from build123d import *

# Parameters (mm, degrees)
SKETCH_1_W                   = 35
SKETCH_1_H                   = 150
EXTRUDE_1_DEPTH              = 4
HOLE_WIZARD_M3_1_D           = 3.4
HOLE_WIZARD_M3_1_CSINK_D     = 6.72
HOLE_WIZARD_M3_1_CSINK_ANGLE = 90


with BuildPart() as part:
    # 草图1 → 凸台-拉伸1 (new body)
    with BuildSketch(Plane.XY):
        Rectangle(SKETCH_1_W, SKETCH_1_H)
    extrude(amount=EXTRUDE_1_DEPTH)

    # M3 六角凹锥坑螺钉的锥形沉头孔1 (through all)
    with Locations(Plane(origin=(-10.25, -35, 4), x_dir=(1, 0, 0), z_dir=(0, 0, 1))):
        with Locations((0, 0), (20.5, 0), (20.5, -30), (0, -30), (0, 100), (20.5, 100), (20.5, 70), (0, 70)):
            CounterSinkHole(HOLE_WIZARD_M3_1_D / 2, HOLE_WIZARD_M3_1_CSINK_D / 2, counter_sink_angle=HOLE_WIZARD_M3_1_CSINK_ANGLE)


solid = part.part
The listing builds one solid part. Answer for the finished solid, in the listing's coordinates (mm). Round coordinates to 2 decimals unless told otherwise and drop trailing zeros. Write each loop counter-clockwise with the first axis right and the second up, starting at its lowest first coordinate (ties: lowest second). Pieces come first, ordered by that corner, then holes. Notation, with made-up numbers: M 80,-26.5 L 136,-26.5 A24 cw 136,-13.5 Z; hole C 84,42.5 d2. An arc over 180 degrees is marked long. Write each question's results on one line, items separated by ' | '. Start each with the question number.
Item 1: A cutting plane is placed at B-B on z = 3.2. State how many separate pieces and enclosed holes the cut face has, and give its area (3 significant figures).
Item 2: Straight lines are drawn through the part: L1, parallel to Y at x = 10.25, z = 1; L2, parallel to X at y = -35, z = 1.5; L3, parallel to X at y = 64, z = 2.7. For each, find the intervals that lie inside material, in ascending order. Write a range as [from, to].
Item 3: Flat-ended cylindrical pins translate along their axes: pin 1 Ø5.5 at (x, y) = (10.25, 65) entering from +Z; pin 2 Ø3 at (x, y) = (10.25, 35) entering from -Z; pin 3 Ø4.5 at (x, y) = (-10.25, 65) entering from +Z. Find the tip coordinate at first contact, or state that the pin passes through.
Item 4: For a pull along X with two mould halves and no side action, classify faces 1 (the face through (0, 1, 4)), 2 (the face through (8.63, 65.51, 1.15)), 3 (the face through (-17.5, -1, 2)) as pulls with the +X half, pulls with the -X half, needs draft (parallel to the pull), parting line crosses it, or undercut.
Item 5: A cutting plane is placed at A-A on y = -65. Write down the section's boundary in (x, z).
Item 6: A cutting plane is placed at C-C on x = 10.25. Write down the section's boundary in (y, z).
Check sheet entries:
1) separate pieces: 1 | enclosed holes: 8 | area: 5,090 mm²
2) L1: [-75, -66.7], [-63.3, -36.7], [-33.3, 33.3], [36.7, 63.3], [66.7, 75] | L2: [-17.5, -11.95], [-8.55, 8.55], [11.95, 17.5] | L3: [-17.5, -12.05], [-8.45, 8.45], [12.05, 17.5]
3) pin 1: z = 3.39 | pin 2: through | pin 3: z = 2.89
4) face 1: needs draft | face 2: undercut | face 3: pulls with the -X half
5) outline: M -17.5,0 L -11.95,0 L -11.95,2.34 L -13.61,4 L -17.5,4 Z; M -8.55,0 L 8.55,0 L 8.55,2.34 L 6.89,4 L -6.89,4 L -8.55,2.34 Z; M 11.95,0 L 17.5,0 L 17.5,4 L 13.61,4 L 11.95,2.34 Z
6) outline: M -75,0 L -66.7,0 L -66.7,2.34 L -68.36,4 L -75,4 Z; M -63.3,0 L -36.7,0 L -36.7,2.34 L -38.36,4 L -61.64,4 L -63.3,2.34 Z; M -33.3,0 L 33.3,0 L 33.3,2.34 L 31.64,4 L -31.64,4 L -33.3,2.34 Z; M 36.7,0 L 63.3,0 L 63.3,2.34 L 61.64,4 L 38.36,4 L 36.7,2.34 Z; M 66.7,0 L 75,0 L 75,4 L 68.36,4 L 66.7,2.34 Z
